Could you check a few things on this drawing? It's one solid part, dimensions in mm from its lowest x, y, z. Give positions to 0.01 mm unless a question says otherwise; leave off trailing zeros. Loops run counter-clockwise (first coordinate to the right, second up) from the corner with the lowest first, then second, coordinate; pieces in that order, holes last. Notation, with made-up numbers: (15, -25) - (58, -25) arc R14 ccw to (58, 1) - close; hole circle Ø1 at (84, 40). An arc over 180 degrees is marked (long way). Write item = value, one per line.
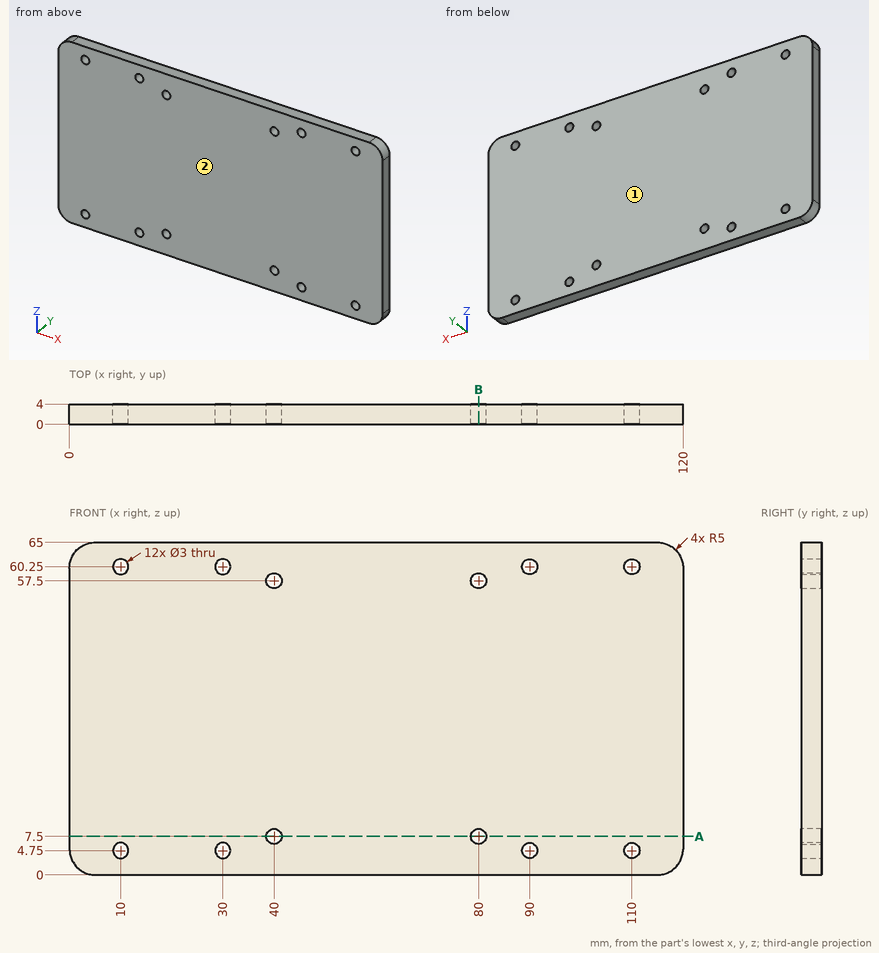
Q1. We'd pull the mould along Y, two halves only. Please class the marked faces 1 and 2: released by +Y, released by -Y, zero draft, split by the parting line, or undercut.
Output:
face_1 = released by +Y
face_2 = released by -Y
Q2. I need wall thicknesses on L1, parallel to Z at x = 10, y = 0.95; L2, parallel to X at y = 1.1, z = 60.25; L3, parallel to Z at x = 80, y = 3.15. Which ranges of each line are inside material? Lowest first, please.
Output:
L1 = 0 to 3.25, 6.25 to 58.75, 61.75 to 65
L2 = 0.01 to 8.5, 11.5 to 28.5, 31.5 to 88.5, 91.5 to 108.5, 111.5 to 119.99
L3 = 0 to 6, 9 to 56, 59 to 65
Q3. Imagine slicing it at B-B, the plane x = 80. Write out the boundary of the cut face in (y, z).
Output:
outline = (0, 0) - (4, 0) - (4, 6) - (0, 6) - close; (0, 9) - (4, 9) - (4, 56) - (0, 56) - close; (0, 59) - (4, 59) - (4, 65) - (0, 65) - close
Q4. Imagine slicing it at A-A, the plane z = 7.5. Write out the boundary of the cut face in (x, y), then the cut area to 3 significant figures.
Output:
outline = (0, 0) - (38.5, 0) - (38.5, 4) - (0, 4) - close; (41.5, 0) - (78.5, 0) - (78.5, 4) - (41.5, 4) - close; (81.5, 0) - (120, 0) - (120, 4) - (81.5, 4) - close
area = 456 mm2
